The listing builds one solid part. Answer for the finished solid, in the listing's coordinates (mm). A direction names the side the tool comes from. Give positions to 0.01 mm unless a question says otherwise; leave off trailing zeros. Loops run counter-clockwise (first coordinate to the right, second up) from the corner with the lowest first, then second, coordinate; pieces in that order, holes last.
Item 1: Consider line 1 along X through (y, z) = (574, 929.5); line 2 along Y through (x, z) = (-581, 647); line 3 along Y through (x, z) = (-607.5, 843). Determine where each line is inside the solid, lowest interval first.
Item 2: Section C-C, the plane z = 354.5 is taken. Give the vertices of the cut face in (x, y).
Item 3: The mould has two halves that part along X. Classify faces 1 (the face through (-570, 590, 516)), 2 (the face through (-590, 570, 516)), 3 (the face through (-573, 590, 531)), 4 (the face through (-590, 607, 516)): pulls with the +X half, pulls with the -X half, needs draft (parallel to the pull), parting line crosses it, or undercut.
Item 4: Section A-A, the plane y = 600 is taken. Give the vertices of the cut face in (x, z).
Item 5: A tool of negligible diameter and unlimited length cuts with its end or side. For faces 5 (the face through (-607, 590, 531)), 6 (the face through (-610, 590, 516)), from which of +Z, -Z, +X, -X, +Y, -Y can it reach the whole face along a straight path? Write none if from no direction.
Item 6: Section B-B, the plane x = -598 is taken. Give the vertices of the cut face in (y, z).
from build123d import *

# Parameters (mm, degrees)
SKETCH1_W           = 40
SKETCH1_H           = 40
BOSS_EXTRUDE1_DEPTH = 1047
FILLET1_R           = 3
SHELL1_START        = -607
SHELL1_OUTLINE_W    = 34
SHELL1_OUTLINE_H    = 1047
SHELL1_DEPTH        = 34


# Read off the part's stored shape, not the designer's step: Shell1
with BuildPart() as part:
    # Sketch1 → Boss-Extrude1 (new body)
    with BuildSketch(Plane.XY):
        with Locations((-590, 590)):
            Rectangle(SKETCH1_W, SKETCH1_H)
    extrude(amount=BOSS_EXTRUDE1_DEPTH)

    # Fillet1
    fillet1_edges = [part.edges().sort_by_distance(p)[0] for p in [
        (-610, 570, 523.5),
        (-570, 570, 523.5),
        (-570, 610, 523.5),
        (-610, 610, 523.5),
    ]]
    fillet(fillet1_edges, radius=FILLET1_R)

    # Shell1 outline → Shell1 (cut)
    with BuildSketch(Plane.YZ.offset(SHELL1_START)):
        with Locations((590, 523.5)):
            Rectangle(SHELL1_OUTLINE_W, SHELL1_OUTLINE_H)
    extrude(amount=SHELL1_DEPTH, mode=Mode.SUBTRACT)


solid = part.part
Worked answers:
1. line 1: x = -610 to -607, -573 to -570
1. line 2: y = 570 to 573, 607 to 610
1. line 3: y = 570.04 to 609.96
2. outline: (-610, 573) arc R3 ccw to (-607, 570) - (-573, 570) arc R3 ccw to (-570, 573) - (-570, 607) arc R3 ccw to (-573, 610) - (-607, 610) arc R3 ccw to (-610, 607) - close; hole (-607, 573) - (-573, 573) - (-573, 607) - (-607, 607) - close
3. face 1: pulls with the +X half
3. face 2: needs draft
3. face 3: undercut
3. face 4: undercut
4. outline: (-610, 0) - (-607, 0) - (-607, 1047) - (-610, 1047) - close; (-573, 0) - (-570, 0) - (-570, 1047) - (-573, 1047) - close
5. face 5: +Z, -Z
5. face 6: +Z, -Z, -X, +Y, -Y
6. outline: (570, 0) - (573, 0) - (573, 1047) - (570, 1047) - close; (607, 0) - (610, 0) - (610, 1047) - (607, 1047) - close
